The model under review builds one solid part; all positions refer to its coordinate system, in mm. Face numbers are marked on the shaded views. A direction names the side the tool comes from. Round coordinates to 2 decimals unless told otherwise and drop trailing zeros. Write each loop counter-clockwise with the first axis right and the second up, starting at its lowest first coordinate (ties: lowest second). Pieces come first, ordered by that corner, then holes. Notation, with made-up numbers: (-9, 29.5) - (47, 29.5) arc R24 cw to (47, 51.5) - close; hole circle Ø11 at (89.25, 11). An arc over 180 degrees is marked (long way). Return JSON: item names as keys, results as strings.
from build123d import *

# Parameters (mm, degrees)
SKETCH2_R           = 2.5
BOSS_EXTRUDE1_DEPTH = 35.5
SKETCH4_W           = 7
SKETCH4_H           = 8
BOSS_EXTRUDE4_DEPTH = 5


with BuildPart() as part:
    # Sketch2 → Boss-Extrude1 (new body)
    with BuildSketch(Plane.XY):
        Circle(SKETCH2_R)
    extrude(amount=BOSS_EXTRUDE1_DEPTH)

    # Sketch4 → Boss-Extrude4 (add)
    with BuildSketch(Plane(origin=(0, 0, 0), x_dir=(-1, 0, 0), z_dir=(0, 0, -1))):
        Rectangle(SKETCH4_W, SKETCH4_H)
    extrude(amount=-BOSS_EXTRUDE4_DEPTH)


solid = part.part
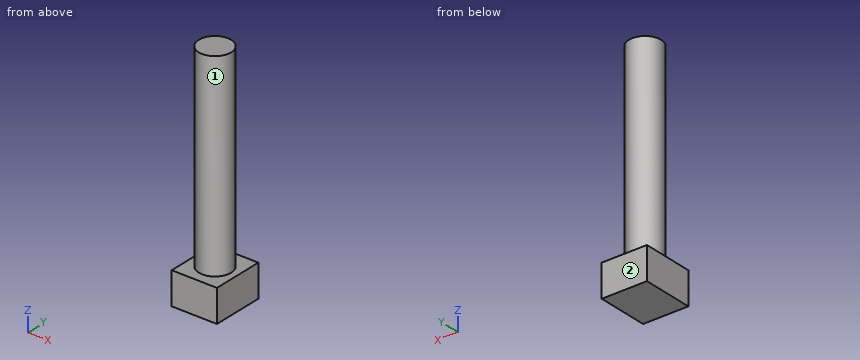
(1) Add section B-B (x = -2). Write out the cut boundary in (y, z), plus the area to 4 significant figures.
Filled in:
{"outline": "(-4, 0) - (4, 0) - (4, 5) - (1.5, 5) - (1.5, 35.5) - (-1.5, 35.5) - (-1.5, 5) - (-4, 5) - close", "area": "131.5 mm2"}
(2) Add section C-C (z = 18.5). Write out the cut boundary in (x, y).
Filled in:
{"outline": "circle Ø5 at (0, 0)"}
(3) Add section D-D (x = 3). Write out the cut boundary in (y, z), plus the area to 3 significant figures.
Filled in:
{"outline": "(-4, 0) - (4, 0) - (4, 5) - (-4, 5) - close", "area": "40.0 mm2"}
(4) Clearance check with flat-ended pins moving along their axes: pin 1 Ø4 at (y, z) = (-2, 24) entering from +X; pin 2 Ø2 at (x, z) = (-1.5, 6.5) entering from +Y. State where each tip first meets the part, or that it passes through.
Filled in:
{"pin 1": "stops at x = 2.5", "pin 2": "stops at y = 2.45"}
(5) Add section A-A (y = -1.5). Write out the cut boundary in (x, z), plus the area to 3 significant figures.
Filled in:
{"outline": "(-3.5, 0) - (3.5, 0) - (3.5, 5) - (2, 5) - (2, 35.5) - (-2, 35.5) - (-2, 5) - (-3.5, 5) - close", "area": "157 mm2"}
(6) Wall thickness on line 1 (Z direction, x = 3, y = 0); line 2 (X direction, y = 0, z = 9); line 3 (X direction, y = 1, z = 7.5): over which ranges is each line inside the solid? List them lowest first.
Filled in:
{"line 1": "z = 0 to 5", "line 2": "x = -2.5 to 2.5", "line 3": "x = -2.29 to 2.29"}
(7) For the marked faces 1 and 2, list the 3-axis set-ups (+Z, -Z, +X, -X, +Y, -Y) from which the entire face can be reached by the end or side of a thin tool; tool diameter is ignored.
Filled in:
{"face 1": "+Z", "face 2": "+Z, -Z, +X, -X, +Y"}
